Answer from the drawing. Dimensions are ordinates in mm from the lowest x, y and z of the part. A direction names the side the tool comes from. Round coordinates to 2 decimals unless told otherwise and drop trailing zeros. Write each loop counter-clockwise with the first axis right and the second up, starting at its lowest first coordinate (ties: lowest second). Pieces come first, ordered by that corner, then holes. Notation, with made-up numbers: (25.25, 25.5) - (56.25, 25.5) arc R14 cw to (56.25, 29.5) - close; hole circle Ø6 at (71, 16.25). An arc over 180 degrees is marked (long way). Answer as CSV lines item,"result". Start each with the question number.
1) Consider line 1 along Y through (x, z) = (17.5, 7.75); line 2 along Y through (x, z) = (28.5, 6.5) (1 decimal); line 3 along X through (y, z) = (19, 13) (1 decimal). Determine where each line is inside the solid, lowest interval first.
2) Find section B-B on y = 43. State how many separate pieces and enclosed holes the cut face has.
3) Each of these flat-tipped pins is pushed along its axis until it touches: pin 1 (5 mm diameter, centred on x = 17, y = 27.5, fed in from +Z); pin 2 (6 mm diameter, centred on y = 43.5, z = 4, fed in from +X); pin 3 (1.6 mm diameter, centred on x = 24, z = 4.5, fed in from +Y); pin 4 (8 mm diameter, centred on y = 41.95, z = 7.57, fed in from +X). Where does it stop, or does it pass through?
4) Which of the six approach directions +Z, -Z, +X, -X, +Y, -Y give full straight-line access (tool end or side, diameter ignored) to the marked faces 3, 4 and 5?
5) Find section D-D on x = 32.5. Determine the outline of the cut face in (y, z) (1 decimal), then the cut area to 3 significant figures.
6) For a pull along Y with two mould halves and no side action, classify the marked faces 1 and 2 as +Y half, -Y half, draft (parallel to the pull), parting line (faces both ways), or undercut.
7) Find section A-A on x = 19. Determine the outline of the cut face in (y, z).
8) Find section C-C on z = 2. Determine the outline of the cut face in (x, y), then the cut area to 3 significant figures.
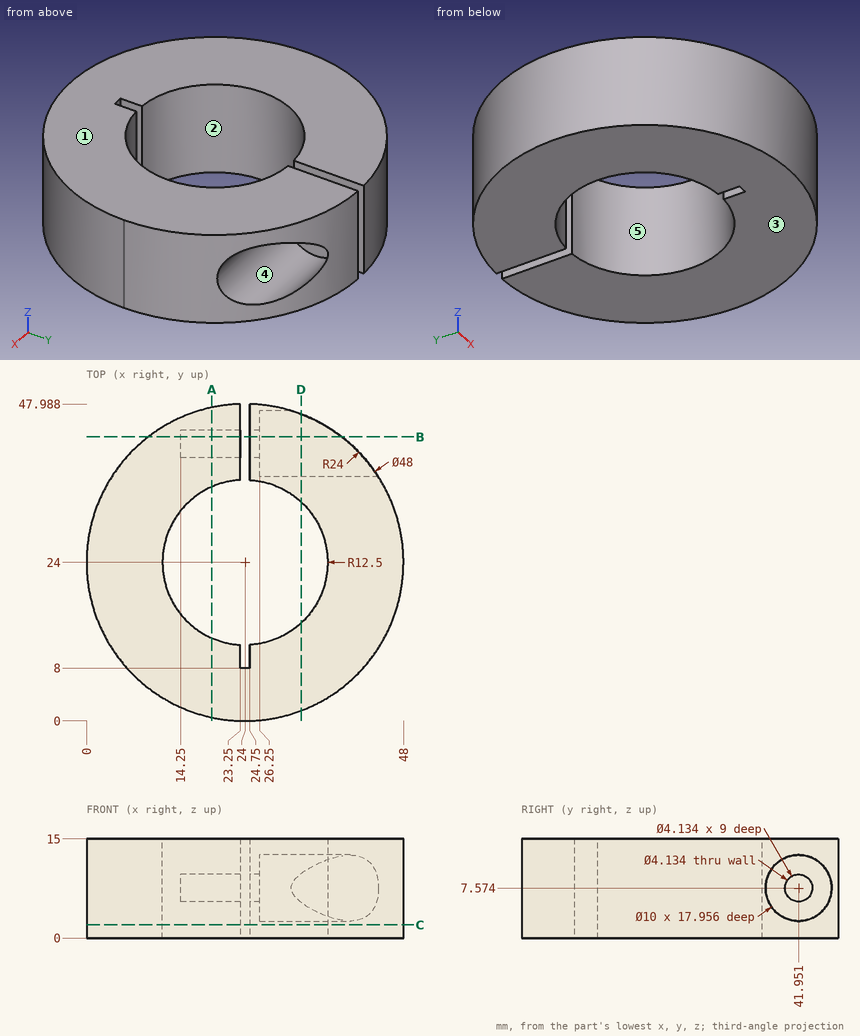
Check values:
1,line 1,"y = 0.9 to 13.32, 34.68 to 39.89, 44.01 to 47.1"
1,line 2,"y = 0.4 to 12.3, 35.7 to 37.1, 46.8 to 47.6"
1,line 3,"x = 0.5 to 12.5, 35.5 to 47.5"
2,separate pieces,"3"
2,enclosed holes,"0"
3,pin 1,"passes through"
3,pin 2,"stops at x = 41.15"
3,pin 3,"stops at y = 47.99"
3,pin 4,"stops at x = 26.25"
4,face 3,"-Z, +X, -X, +Y, -Y"
4,face 4,"+X"
4,face 5,"+Z, -Z"
5,outline,"(1.6, 0) - (14.8, 0) - (14.8, 15) - (1.6, 15) - close; (33.2, 0) - (46.4, 0) - (46.4, 5.4) arc R5 cw (long way) to (46.4, 9.8) - (46.4, 15) - (33.2, 15) - close"
5,area,"321 mm^2"
6,face 1,"draft"
6,face 2,"undercut"
7,outline,"(0.53, 0) - (12.54, 0) - (12.54, 15) - (0.53, 15) - close; (35.46, 0) - (47.47, 0) - (47.47, 15) - (35.46, 15) - close; hole circle Ø4.13 at (41.95, 7.57)"
8,outline,"(23.25, 8) - (23.25, 11.52) arc R12.5 cw to (23.25, 36.48) - (23.25, 47.99) arc R24 ccw (long way) to (24.75, 47.99) - (24.75, 36.48) arc R12.5 cw to (24.75, 11.52) - (24.75, 8) - close"
8,area,"1,300 mm^2"
